Geometry: final body of the model. Coordinates: model frame, mm. A direction names the side the tool comes from. Give positions to 0.01 mm unless a question says otherwise; leave off trailing zeros. Write each loop counter-clockwise with the first axis right and the second up, starting at its lowest first coordinate (ties: lowest second). Pieces come first, ordered by that corner, then holes. Notation, with made-up numbers: M 8.5,87.5 L 22.5,87.5 A15 ccw 22.5,92.5 Z; hole C 3,85 d9. An arc over 180 degrees is marked long. Use a Markdown table: item, result. Add a question column.
(1) Material intervals for L1, parallel to Z at x = -29, y = 7; L2, parallel to Z at x = -19, y = 14; L3, parallel to Z at x = -9.5, y = 14.5, sorted ascending.
(2) Reachability of faces 1 (the flat face through (-16, 0, 132)), 2 (the flat face through (-16, 19.05, 471)), 3 (the flat face through (-16, 12.7, 471)) from +Z, -Z, +X, -X, +Y, -Y: full face, straight path, thin tool, end or side. Return the list, or none.
(3) Cut plane A-A (y = 7). Output: boundary loops of the cut face in (x, z), plus the area to 3 significant figures.
(4) Pin query (flat end, axial travel): pin 1 Ø5 at (y, z) = (15.5, 471.5) entering from +X; pin 2 Ø3 at (y, z) = (16, 465.5) entering from -X; pin 3 Ø9.5 at (x, y) = (-21.5, 23) entering from +Z. Return the tip coordinate at first contact, or that it passes through.
```python
from build123d import *

# Parameters (mm, degrees)
F0_W     = 31.75
F0_H     = 666.75
F1_DEPTH = 31.75
F2_W     = 19.05
F2_H     = 6.35
F3_DEPTH = 25.4
F4_R     = 9.52499
F5_R     = 3.81
F6_DEPTH = 6.35


# Not quite as in the source:
# - a fillet or chamfer is up to 0.001 mm smaller than in the source, because OpenCascade refuses the exact size


with BuildPart() as f1:
    # F0 (on Front) → F1 (new body)
    with BuildSketch(Plane.XZ):
        with Locations((-15.875, 127.5886728781)):
            Rectangle(F0_W, F0_H)
    extrude(amount=-F1_DEPTH)

    # F2 (on face) → F3 (join)
    with BuildSketch(Plane.XY.offset(460.9636728781)):
        with Locations((-15.875, 15.875)):
            Rectangle(F2_W, F2_H)
    extrude(amount=F3_DEPTH)

    # F4 (radius 9.525 in the source; OpenCascade refuses exactly that, so slightly less here)
    f4_edges = [f1.edges().sort_by_distance(p)[0] for p in [
        (-6.35, 15.875, 486.363673),
        (-25.4, 15.875, 486.363673),
    ]]
    fillet(f4_edges, radius=F4_R)

    # F5 (on face) → F6 (cut)
    with BuildSketch(Plane.XZ.offset(-12.7)):
        with Locations((-15.875, 476.8386728781)):
            Circle(F5_R)
    extrude(amount=-F6_DEPTH, mode=Mode.SUBTRACT)


solid = f1.part
```
Answer list:
| question | item | result |
|---|---|---|
| 1 | L1 | -205.79 to 460.96 |
| 1 | L2 | -205.79 to 474.66, 479.02 to 485.84 |
| 1 | L3 | -205.79 to 483.92 |
| 2 | face 1 | +Z, -Z, +X, -X, -Y |
| 2 | face 2 | +Z, +X, -X, +Y |
| 2 | face 3 | +Z, +X, -X, -Y |
| 3 | outline | M -31.75,-205.79 L 0,-205.79 L 0,460.96 L -31.75,460.96 Z |
| 3 | area | 21,200 mm² |
| 4 | pin 1 | x = -6.35 |
| 4 | pin 2 | x = -25.4 |
| 4 | pin 3 | z = 485.88 |
